The listing builds one solid part. Answer for the finished solid, in the listing's coordinates (mm). Coordinates: 2 decimals unless noted, no trailing zeros. Order: outer loops, then holes, each group sorted by start corner. A loop starts at its lowest first (then second) coordinate and runs counter-clockwise, first axis right, second up. Notation, with made-up numbers: (40, 85) - (79, 85) arc R13 ccw to (79, 95) - close; hole circle Ø1 at (34, 3). An arc over 180 degrees is marked (long way). Use one line per item in the form item = value. Start each with the question number.
Item 1: Section D-D, the plane x = 6 is taken. Write down the section's boundary in (y, z).
Item 2: Section A-A, the plane z = 0 is taken. Write down the section's boundary in (x, y).
Item 3: Section B-B, the plane x = 0 is taken. Write down the section's boundary in (y, z).
Item 4: Consider line 1 along X through (y, z) = (3.25, 0); line 2 along Z through (x, y) = (-8.5, 3); line 3 along X through (y, z) = (9.5, -12). Determine where each line is inside the solid, lowest interval first. Write a range as [from, to].
Item 5: The mould has two halves that part along X. Classify faces 1 (the cylindrical face through (-17.36, 6.26, -3.85)), 2 (the cylindrical face through (-12.086, 6.439, 4.355)): released by +X, released by -X, zero draft, split by the parting line, or undercut.
Item 6: Section C-C, the plane y = 2 is taken. Count the separate pieces of the cut face and the enclosed holes in it, and give its area (3 significant figures).
Item 7: Each of these flat-tipped pins is pushed along its axis until it touches: pin 1 Ø2 at (x, z) = (-2.5, -12.5) entering from -Y; pin 2 Ø5 at (x, y) = (10.5, 4) entering from -Z; pin 3 Ø3 at (x, y) = (8, 2) entering from -Z; pin 4 Ø3 at (x, y) = (-6.5, 2.5) entering from -Z. Where does it stop, or does it pass through?
from build123d import *

# Parameters (mm, degrees)
SKETCH1_R           = 17.78
SKETCH1_R_2         = 7.9375
BOSS_EXTRUDE1_DEPTH = 12.7
CUT_EXTRUDE1_DEPTH  = 29.169962726
CIRPATTERN1_COUNT   = 6


with BuildPart() as part:
    # Sketch1 → Boss-Extrude1 (new body)
    with BuildSketch(Plane(origin=(0, 0, 0), x_dir=(1, 0, 0), z_dir=(0, 1, 0))):
        with Locations(Location((0, 0, 0), (0, 0, 270))):
            Circle(SKETCH1_R)
        with Locations(Location((0, 0, 0), (0, 0, 270))):
            Circle(SKETCH1_R_2, mode=Mode.SUBTRACT)
    extrude(amount=BOSS_EXTRUDE1_DEPTH)

    # Sketch2 → Cut-Extrude1 (cut, through all)
    with BuildSketch(Plane(origin=(0, 12.7, 0), x_dir=(1, 0, 0), z_dir=(0, 1, 0))):
        with BuildLine():
            ThreePointArc((6.615, 14.293504644), (7.875, 13.63990011), (9.071038131, 12.875510368))
            ThreePointArc((9.071038131, 12.875510368), (9.856087957, 8.346857503), (5.327435093, 7.561807676))
            ThreePointArc((5.327435093, 7.561807676), (4.625, 8.010734985), (3.885, 8.394597965))
            ThreePointArc((3.885, 8.394597965), (2.300546661, 12.709051305), (6.615, 14.293504644))
        make_face()
    cut_extrude1 = extrude(amount=-CUT_EXTRUDE1_DEPTH, mode=Mode.SUBTRACT)

    # CirPattern1: Cut-Extrude1 ×6 about axis
    cirpattern1_axis = Axis((0, 0, 0), (0, 1, 0))
    for i in range(1, CIRPATTERN1_COUNT):
        add(cut_extrude1.rotate(cirpattern1_axis, i * 360 / CIRPATTERN1_COUNT), mode=Mode.SUBTRACT)


solid = part.part
Response:
q1.outline = (0, -16.74) - (12.7, -16.74) - (12.7, -14.51) - (0, -14.51) - close; (0, -7.2) - (12.7, -7.2) - (12.7, -5.2) - (0, -5.2) - close; (0, 5.2) - (12.7, 5.2) - (12.7, 7.2) - (0, 7.2) - close; (0, 14.51) - (12.7, 14.51) - (12.7, 16.74) - (0, 16.74) - close
q2.outline = (-17.78, 0) - (-15.75, 0) - (-15.75, 12.7) - (-17.78, 12.7) - close; (-9.25, 0) - (-7.94, 0) - (-7.94, 12.7) - (-9.25, 12.7) - close; (7.94, 0) - (9.25, 0) - (9.25, 12.7) - (7.94, 12.7) - close; (15.75, 0) - (17.78, 0) - (17.78, 12.7) - (15.75, 12.7) - close
q3.outline = (0, -17.78) - (12.7, -17.78) - (12.7, -7.94) - (0, -7.94) - close; (0, 7.94) - (12.7, 7.94) - (12.7, 17.78) - (0, 17.78) - close
q4.line_1 = [-17.78, -15.75], [-9.25, -7.94], [7.94, 9.25], [15.75, 17.78]
q4.line_2 = [-15.62, -13.26], [-7.24, 7.24], [13.26, 15.62]
q4.line_3 = [-13.12, -9.92], [-2.07, 2.07], [9.92, 13.12]
q5.face_1 = split by the parting line
q5.face_2 = undercut
q6.separate_pieces = 1
q6.enclosed_holes = 7
q6.area = 508 mm2
q7.pin_1 = 0
q7.pin_2 = -15.88
q7.pin_3 = -16.55
q7.pin_4 = -17.06
